Build history of the part. All positions in model axes, mm. Give positions to 0.01 mm unless a question says otherwise; leave off trailing zeros. Order: outer loops, then holes, each group sorted by start corner. A loop starts at its lowest first (then second) coordinate and runs counter-clockwise, first axis right, second up. Notation, with made-up numbers: (23.5, -34) - (52.5, -34) arc R3 ccw to (52.5, -30) - close; hole circle Ø1 at (83.5, 33.5). An arc over 180 degrees is marked (long way). Write each question's results on one line, items separated by ' | '. Start each with the question number.
1) Cut at D-D on y = 126. List the corners of the cut face in (x, z).
2) Cut at C-C on y = 184. List the corners of the cut face in (x, z).
3) Cut at B-B on x = 35.5. List the corners of the cut face in (y, z), plus the area to 3 significant figures.
4) Drill centre lines: line 1 along Y through (x, z) = (35, 11.5); line 2 along X through (y, z) = (184, 13); line 3 along X through (y, z) = (74, 12.25). Where is each one in solid material? Low to high. Write a range as from..to.
5) Cut at A-A on y = 16. List the corners of the cut face in (x, z).
6) Drop a flat-ended pin along its axis: pin 1 Ø8 at (x, y) = (-35.5, 16) entering from +Z. Give the stop position or say it passes through.
from build123d import *

# Parameters (mm, degrees)
F0_W     = 400
F0_H     = 200
F0_W_2   = 284
F0_H_2   = 120
F1_DEPTH = 20
F2_D     = 8.8
F4_D     = 13.2
F4_DEPTH = 50
F4_TIP   = 3.9656800856


with BuildPart() as f1:
    # F0 (on Top) → F1 (new body)
    with BuildSketch(Plane.XY):
        with Locations((0, 100)):
            Rectangle(F0_W, F0_H)
        with Locations((0, 100)):
            Rectangle(F0_W_2, F0_H_2, mode=Mode.SUBTRACT)
    extrude(amount=F1_DEPTH)

    # F2 (through all)
    with Locations(Plane(origin=(0, 0, 0), x_dir=(1, 0, 0), z_dir=(0, 0, -1))):
        with Locations((-157, -126), (-157, -74), (-106.5, -16), (-35.5, -16), (35.5, -16), (106.5, -16), (157, -74), (157, -126), (106.5, -184), (35.5, -184), (-35.5, -184), (-106.5, -184)):
            Hole(F2_D / 2)

    # F4
    with Locations(Plane.XZ):
        with Locations((-150, 10), (150, 10), (0, 10)):
            Hole(F4_D / 2, depth=F4_DEPTH)
            with Locations((0, 0, -(F4_DEPTH + F4_TIP / 2))):  # 118° drill point
                Cone(0, F4_D / 2, F4_TIP, mode=Mode.SUBTRACT)


solid = f1.part
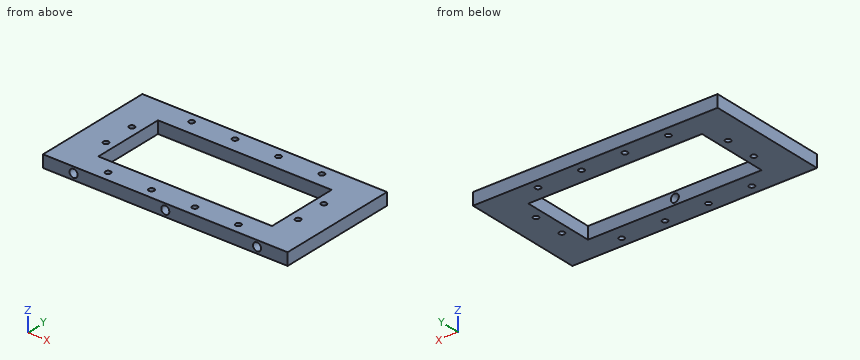
Results:
1) outline: (-200, 0) - (-161.4, 0) - (-161.4, 20) - (-200, 20) - close; (-152.6, 0) - (-142, 0) - (-142, 20) - (-152.6, 20) - close; (142, 0) - (152.6, 0) - (152.6, 20) - (142, 20) - close; (161.4, 0) - (200, 0) - (200, 20) - (161.4, 20) - close
2) outline: (-200, 0) - (-110.9, 0) - (-110.9, 20) - (-200, 20) - close; (-102.1, 0) - (-39.9, 0) - (-39.9, 20) - (-102.1, 20) - close; (-31.1, 0) - (31.1, 0) - (31.1, 20) - (-31.1, 20) - close; (39.9, 0) - (102.1, 0) - (102.1, 20) - (39.9, 20) - close; (110.9, 0) - (200, 0) - (200, 20) - (110.9, 20) - close
3) outline: (0, 0) - (11.6, 0) - (11.6, 20) - (0, 20) - close; (20.4, 0) - (40, 0) - (40, 20) - (20.4, 20) - close; (160, 0) - (179.6, 0) - (179.6, 20) - (160, 20) - close; (188.4, 0) - (200, 0) - (200, 20) - (188.4, 20) - close | area: 1,250 mm^2
4) line 1: 0..11.63, 20.37..40, 160..179.63, 188.37..200 | line 2: -200..-110.9, -102.1..-39.9, -31.1..31.1, 39.9..102.1, 110.9..200 | line 3: -200..-161.4, -152.6..-142, 142..152.6, 161.4..200
5) outline: (-200, 0) - (-110.9, 0) - (-110.9, 20) - (-200, 20) - close; (-102.1, 0) - (-39.9, 0) - (-39.9, 20) - (-102.1, 20) - close; (-31.1, 0) - (31.1, 0) - (31.1, 20) - (-31.1, 20) - close; (39.9, 0) - (102.1, 0) - (102.1, 20) - (39.9, 20) - close; (110.9, 0) - (200, 0) - (200, 20) - (110.9, 20) - close; hole circle Ø13.2 at (-150, 10); hole circle Ø13.2 at (0, 10); hole circle Ø13.2 at (150, 10)
6) pin 1: through
